```python
from build123d import *

# Parameters (mm, degrees)
F1_DEPTH = 25.4


with BuildPart() as f1:
    # F0 (on Front) → F1 (new body)
    with BuildSketch(Plane.XZ):
        with BuildLine():
            Line((385.175922, -833.611421), (385.175922, 0))
            Line((385.175922, 0), (385.175922, 508))
            Line((385.175922, 508), (-376.824078, 508))
            Line((-376.824078, 508), (-376.824078, -833.611421))
            ThreePointArc((-376.824078, -833.611421), (4.175922, -939.8), (385.175922, -833.611421))
        make_face()
        with BuildLine():
            ThreePointArc((4.175922, -126.931327), (-91.267032, 88.313809), (127, 0))
            ThreePointArc((127, 0), (91.267032, -88.313809), (4.175922, -126.931327))
        make_face(mode=Mode.SUBTRACT)
    extrude(amount=F1_DEPTH)


solid = f1.part
```
Input: part model. Units: mm. Frame: model coordinates. Coordinates: 2 decimals unless noted, no trailing zeros. Write each loop counter-clockwise with the first axis right and the second up, starting at its lowest first coordinate (ties: lowest second). Pieces come first, ordered by that corner, then holes. Notation, with made-up numbers: (81, 7.5) -> (95, 7.5) arc R23 ccw to (95, 15.5) -> close; hole circle Ø9 at (14.5, 8). An arc over 180 degrees is marked (long way). Answer as a JSON object with one key per item and string values.
1. First-contact query: P1, Ø2, axis at x = -204.5, y = -16.5, coming from the -Z side. Flat tip, straight axial feed; report the tip coordinate or a pass-through.
Result set:
{"P1": "stops at z = -909.92"}
2. Material intervals for line 1 (Z direction, x = 0, y = -13.25); line 2 (X direction, y = -9.75, z = 0); line 3 (Z direction, x = 99, y = -5), sorted ascending. Write a range as from..to.
Result set:
{"line 1": "z = -939.79..-127, 127..508", "line 2": "x = -376.82..-127, 127..385.18", "line 3": "z = -933.67..-79.55, 79.55..508"}
3. Section A-A on z = 106. Return the cut outline in (x, y), then the cut area to 3 significant figures.
Result set:
{"outline": "(-376.82, -25.4) -> (-69.95, -25.4) -> (-69.95, 0) -> (-376.82, 0) -> close; (69.95, -25.4) -> (385.18, -25.4) -> (385.18, 0) -> (69.95, 0) -> close", "area": "15,800 mm2"}
4. Section D-D on x = -181.5. Return the cut outline in (y, z), then the cut area to 3 significant figures.
Result set:
{"outline": "(-25.4, -916.01) -> (0, -916.01) -> (0, 508) -> (-25.4, 508) -> close", "area": "36,200 mm2"}
5. Section B-B on x = -88. Return the cut outline in (y, z).
Result set:
{"outline": "(-25.4, -934.01) -> (0, -934.01) -> (0, -91.57) -> (-25.4, -91.57) -> close; (-25.4, 91.57) -> (0, 91.57) -> (0, 508) -> (-25.4, 508) -> close"}
6. Section C-C on y = -4.5. Return the cut outline in (x, z).
Result set:
{"outline": "(-376.82, -833.61) arc R736.6 ccw to (385.18, -833.61) -> (385.18, 508) -> (-376.82, 508) -> close; hole circle Ø254 at (0, 0)"}
